from build123d import *

# Parameters (mm, degrees)
SKETCH1_W                            = 190.5
SKETCH1_H                            = 76.2
BOSS_EXTRUDE1_DEPTH                  = 50.8
FILLET1_R                            = 1.524
F_41_64_0_64063_DIAMETER_HOLE1_D     = 16.272002
F_41_64_0_64063_DIAMETER_HOLE1_DEPTH = 26.162
F_1_2_0_5_DIAMETER_HOLE1_D           = 13.4874
CUT_EXTRUDE1_DEPTH                   = 12.7


with BuildPart() as part:
    # Sketch1 → Boss-Extrude1 (new body)
    with BuildSketch(Plane.XY):
        Rectangle(SKETCH1_W, SKETCH1_H)
    extrude(amount=BOSS_EXTRUDE1_DEPTH)

    # Fillet1
    fillet1_edges = [part.edges().sort_by_distance(p)[0] for p in [
        (0, 38.1, 50.8),
        (0, 38.1, 0),
        (0, -38.1, 0),
        (0, -38.1, 50.8),
    ]]
    fillet(fillet1_edges, radius=FILLET1_R)

    # 41/64 (0.64063) Diameter Hole1
    with Locations(Plane.XY.offset(50.8)):
        with Locations((-69.85, 0), (-31.75, 0), (6.35, 0)):
            Hole(F_41_64_0_64063_DIAMETER_HOLE1_D / 2, depth=F_41_64_0_64063_DIAMETER_HOLE1_DEPTH)

    # 1/2 (0.5) Diameter Hole1 (through all)
    with Locations(Plane.XY.offset(50.8)):
        with Locations((60.325, 28.575), (85.725, 28.575), (60.325, -28.575), (85.725, -28.575)):
            Hole(F_1_2_0_5_DIAMETER_HOLE1_D / 2)

    # Sketch7 → Cut-Extrude1 (cut)
    with BuildSketch(Plane.XY.offset(50.8)):
        with BuildLine():
            Line((95.25, 38.1), (44.45, 38.1))
            Line((44.45, 38.1), (44.45, 23.8252))
            ThreePointArc((44.45, 23.8252), (46.309871939, 19.335071939), (50.8, 17.4752))
            Line((50.8, 17.4752), (95.25, 17.4752))
            Line((95.25, 17.4752), (95.25, 38.1))
        make_face()
        with BuildLine():
            Line((50.8, -17.4752), (95.25, -17.4752))
            Line((95.25, -17.4752), (95.25, -38.1))
            Line((95.25, -38.1), (44.45, -38.1))
            Line((44.45, -38.1), (44.45, -23.8252))
            ThreePointArc((44.45, -23.8252), (46.309871939, -19.335071939), (50.8, -17.4752))
        make_face()
    extrude(amount=-CUT_EXTRUDE1_DEPTH, mode=Mode.SUBTRACT)


solid = part.part
The model under review builds one solid part; all positions refer to its coordinate system, in mm. A direction names the side the tool comes from. Give positions to 0.01 mm unless a question says otherwise; leave off trailing zeros. Loops run counter-clockwise (first coordinate to the right, second up) from the corner with the lowest first, then second, coordinate; pieces in that order, holes last. Notation, with made-up numbers: (-13, 59) -> (42, 59) arc R11 cw to (42, 63) -> close; hole circle Ø4 at (89.25, 70.25). An arc over 180 degrees is marked (long way). Put each result on its own line as item: value. Start each with the question number.
1. We need section C-C on x = 6.35. State the section outline as (y, z) points.
2. Wall thickness on probe 1 along X at (y, z) = (-0.5, 44); probe 2 along X at (y, z) = (-32.5, 2); probe 3 along X at (y, z) = (-29.5, 10): over which ranges is each line inside the solid? List them lowest first.
3. Mouldability with a two-part tool opening along Y and no side actions: class faces 4 (the face through (44.45, -31, 45)), 5 (the face through (-70, 0, 24.638)), 6 (the face through (-1, -38.1, 25)) as released by +Y, released by -Y, zero draft, split by the parting line, or undercut.
4. We need section B-B on z = 30. State the section outline as (x, y) points (3 decimals), then the cut area to 3 significant figures.
5. For faces 1 (the face through (46.261, 19.385, 44.539)), 2 (the face through (-39.266, -3.116, 37.536)), 3 (the face through (73, -17.475, 45)), list the 3-axis set-ups (+Z, -Z, +X, -X, +Y, -Y) from which the entire face can be reached by the end or side of a thin tool; tool diameter is ignored.
6. We need section D-D on z = 8.5. State the section outline as (x, y) points (3 decimals).
7. We need section A-A on y = 0. State the section outline as (x, z) points.
8. Clearance check with flat-ended pins moving along their axes: P1, Ø2, axis at x = 54.5, z = 42, coming from the -Y side; P2, Ø4, axis at x = 66.5, z = 46.5, coming from the +Y side; P3, Ø15.5, axis at x = 60.325, y = -28.575, coming from the +Z side. State where each tip first meets the part, or that it passes through.
Determined:
1. outline: (-38.1, 1.52) arc R1.52 ccw to (-36.58, 0) -> (36.58, 0) arc R1.52 ccw to (38.1, 1.52) -> (38.1, 49.28) arc R1.52 ccw to (36.58, 50.8) -> (8.14, 50.8) -> (8.14, 24.64) -> (-8.14, 24.64) -> (-8.14, 50.8) -> (-36.58, 50.8) arc R1.52 ccw to (-38.1, 49.28) -> close
2. probe 1: -95.25 to -77.97, -61.73 to -39.87, -23.63 to -1.77, 14.47 to 95.25
2. probe 2: -95.25 to 54.84, 65.81 to 80.24, 91.21 to 95.25
2. probe 3: -95.25 to 53.65, 67 to 79.05, 92.4 to 95.25
3. face 4: zero draft
3. face 5: undercut
3. face 6: released by -Y
4. outline: (-95.25, -38.1) -> (95.25, -38.1) -> (95.25, 38.1) -> (-95.25, 38.1) -> close; hole circle Ø16.272 at (-69.85, 0); hole circle Ø16.272 at (-31.75, 0); hole circle Ø16.272 at (6.35, 0); hole circle Ø13.487 at (60.325, -28.575); hole circle Ø13.487 at (60.325, 28.575); hole circle Ø13.487 at (85.725, -28.575); hole circle Ø13.487 at (85.725, 28.575)
4. area: 13,300 mm^2
5. face 1: +Z, +X, +Y
5. face 2: +Z
5. face 3: +Z, +X, -Y
6. outline: (-95.25, -38.1) -> (95.25, -38.1) -> (95.25, 38.1) -> (-95.25, 38.1) -> close; hole circle Ø13.487 at (60.325, -28.575); hole circle Ø13.487 at (60.325, 28.575); hole circle Ø13.487 at (85.725, -28.575); hole circle Ø13.487 at (85.725, 28.575)
7. outline: (-95.25, 0) -> (95.25, 0) -> (95.25, 50.8) -> (14.49, 50.8) -> (14.49, 24.64) -> (-1.79, 24.64) -> (-1.79, 50.8) -> (-23.61, 50.8) -> (-23.61, 24.64) -> (-39.89, 24.64) -> (-39.89, 50.8) -> (-61.71, 50.8) -> (-61.71, 24.64) -> (-77.99, 24.64) -> (-77.99, 50.8) -> (-95.25, 50.8) -> close
8. P1: y = -17.48
8. P2: y = 17.48
8. P3: z = 38.1
